```python
from build123d import *

# Parameters (mm, degrees)
SKETCH1_W          = 75
SKETCH1_H          = 6.35
BASE_EXTRUDE_DEPTH = 19.05
CUT_EXTRUDE1_DEPTH = 7.35
SKETCH3_R          = 2.622460094
CUT_EXTRUDE2_DEPTH = 7.35
CHAMFER1_SIZE      = 1.27


with BuildPart() as part:
    # Sketch1 → Base-Extrude (new body)
    with BuildSketch(Plane.XY):
        with Locations((37.5, 3.175)):
            Rectangle(SKETCH1_W, SKETCH1_H)
    extrude(amount=BASE_EXTRUDE_DEPTH)

    # Sketch2 → Cut-Extrude1 (cut, through all)
    with BuildSketch(Plane(origin=(0, 6.35, 0), x_dir=(-1, 0, 0), z_dir=(0, 1, 0))):
        with BuildLine():
            Line((-70.3645, 5.67551708), (-70.3645, 13.37448292))
            ThreePointArc((-70.3645, 13.37448292), (-59.252, 9.525), (-70.3645, 5.67551708))
        make_face()
    extrude(amount=-CUT_EXTRUDE1_DEPTH, mode=Mode.SUBTRACT)

    # Sketch3 → Cut-Extrude2 (cut, through all)
    with BuildSketch(Plane(origin=(0, 6.35, 0), x_dir=(-1, 0, 0), z_dir=(0, 1, 0))):
        with Locations((-9.525, 9.525)):
            Circle(SKETCH3_R)
    extrude(amount=-CUT_EXTRUDE2_DEPTH, mode=Mode.SUBTRACT)

    # Chamfer1
    chamfer1_edges = [part.edges().sort_by_distance(p)[0] for p in [
        (37.5, 0, 19.05),
        (37.5, 0, 0),
        (37.5, 6.35, 0),
        (37.5, 6.35, 19.05),
        (0, 0, 9.525),
        (75, 0, 9.525),
        (75, 6.35, 9.525),
        (0, 6.35, 9.525),
    ]]
    chamfer(chamfer1_edges, length=CHAMFER1_SIZE)


solid = part.part
```
Build history of the part. All positions in model axes, mm. Round coordinates to 2 decimals unless told otherwise and drop trailing zeros. Loops run counter-clockwise (first coordinate to the right, second up) from the corner with the lowest first, then second, coordinate; pieces in that order, holes last.
Item 1: Saw through at B-B (z = 4.5). List the corners of the cut face in (x, y), then the cut area to 3 significant figures.
Item 2: Saw through at D-D (x = 60). List the corners of the cut face in (y, z), then the cut area to 3 significant figures.
Item 3: Drill centre lines: line 1 along X through (y, z) = (6, 9); line 2 along X through (y, z) = (3, 8.25); line 3 along Z through (x, y) = (67.5, 4.5). Where is each one in solid material? Low to high.
Item 4: Two-plate mould, pull along Z, no slides. Class faces 1 (the face through (59.256, 3.219, 9.741)), 2 (the face through (70.364, 3, 9)), 3 (the face through (74.37, 5.71, 9.39)), 4 (the face through (36.98, 5.71, 18.42)): released by +Z, released by -Z, zero draft, split by the parting line, or undercut.
Item 5: Saw through at C-C (y = 2). State how many separate pieces and enclosed holes the cut face has, then the cut area to 3 significant figures.
Item 6: Saw through at A-A (x = 37.5). List the corners of the cut face in (y, z).
Item 7: Pin check, flat tips, straight feed: P1, Ø4, axis at x = 9.525, z = 9.525, coming from the -Y side; P2, Ø3, axis at x = 48, z = 5.5, coming from the -Y side. Stop position of each tip, or through.
Worked answers:
1. outline: (0, 1.27) - (1.27, 0) - (61.8, 0) - (61.8, 6.35) - (1.27, 6.35) - (0, 5.08) - close; (69.15, 0) - (73.73, 0) - (75, 1.27) - (75, 5.08) - (73.73, 6.35) - (69.15, 6.35) - close
1. area: 426 mm2
2. outline: (0, 1.27) - (1.27, 0) - (5.08, 0) - (6.35, 1.27) - (6.35, 6.57) - (0, 6.57) - close; (0, 12.48) - (6.35, 12.48) - (6.35, 17.78) - (5.08, 19.05) - (1.27, 19.05) - (0, 17.78) - close
2. area: 80.2 mm2
3. line 1: x = 0.92 to 6.96, 12.09 to 59.27, 70.36 to 74.08
3. line 2: x = 0 to 7.23, 11.82 to 59.38, 70.36 to 75
3. line 3: z = 0 to 3.64, 15.41 to 19.05
4. face 1: undercut
4. face 2: undercut
4. face 3: zero draft
4. face 4: released by +Z
5. separate pieces: 1
5. enclosed holes: 2
5. area: 1,290 mm2
6. outline: (0, 1.27) - (1.27, 0) - (5.08, 0) - (6.35, 1.27) - (6.35, 17.78) - (5.08, 19.05) - (1.27, 19.05) - (0, 17.78) - close
7. P1: passes through
7. P2: stops at y = 0
